Here's how the part is built. I have some questions about the finished solid (model axes, mm). A direction names the side the tool comes from. Coordinates: 2 decimals unless noted, no trailing zeros. Write each loop counter-clockwise with the first axis right and the second up, starting at its lowest first coordinate (ties: lowest second). Pieces come first, ordered by that corner, then holes. Notation, with made-up numbers: (-2.5, 84.25) - (1.5, 84.25) arc R20 cw to (1.5, 91.25) - close; hole circle Ø2 at (50.5, 71). An arc over 180 degrees is marked (long way). Answer in a Markdown table with one row per item. Add a question column.
Item 1: Imagine slicing it at B-B (z = -15). Please give me the cut outline in (x, y).
Item 2: We'd pull the mould along X, two halves only. Please class faces 5 (the face through (11, 37.369, -15)), 6 (the face through (30.322, 22, -15)), 7 (the face through (-22.678, 19, -17)): +X half, -X half, draft (parallel to the pull), parting line (faces both ways), or undercut.
Item 3: Which directions (+Z, -Z, +X, -X, +Y, -Y) give clear straight access to the entire face, cutting with the end or side of a thin tool? Please do faces 1 (the face through (25.322, 20, -17)), 2 (the face through (40, 6.369, -19)), 3 (the face through (-38, 6.369, -19)), 4 (the face through (-8.679, 33, -11)).
Item 4: Imagine slicing it at A-A (y = 31). Please give me the cut outline in (x, z).
Item 5: Imagine slicing it at D-D (x = 4). Please give me the cut outline in (y, z), plus the area to 3 significant figures.
Item 6: I'm going to push flat-ended pins straight in: pin 1 (5.5 mm diameter, centred on y = 25.5, z = -8.5, fed in from -X); pin 2 (12 mm diameter, centred on x = 16, y = 25.5, fed in from -Z); pin 3 (4.5 mm diameter, centred on x = 40.32, z = -15, fed in from +Y); pin 4 (7.5 mm diameter, centred on y = 16.5, z = -19.5, fed in from +X). Where does each tip first touch, or does it pass through?
Item 7: Imagine slicing it at C-C (y = 20.5). Please give me the cut outline in (x, z).
Item 8: If I drill on probe 1 along X at (y, z) = (31.5, -11); probe 2 along Y at (x, z) = (0.5, -22.5); probe 3 along Y at (x, z) = (-28, -25), over which ranges is the centre line in solid material (lowest first)? Write a range as from..to.
from build123d import *

# Parameters (mm, degrees)
F1_DEPTH = 30
F0_R     = 6.25
F2_DEPTH = 5
F3_W     = 5
F3_H     = 30
F4_DEPTH = 20
F5_W     = 5
F5_H     = 30
F6_DEPTH = 20
F7_R     = 2.5
F8_DEPTH = 25


# Not quite as in the source:
# - a feature names something its author has since deleted; it is built from what else it names


with BuildPart() as f1:
    # F0 (on Top) → F1 (new body)
    with BuildSketch(Plane.XY):
        Polygon((25.3224579843, 32.3690634753), (25.3224579843, 6.3690634753), (30.3224579843, 6.3690634753), (30.3224579843, 37.3690634753), (-8.6790506474, 37.3690634753), (-8.6790506474, 32.3690634753), align=None)
        Polygon((-22.6775420157, 6.3690634753), (-22.6775420157, 32.3690634753), (-21.1775420157, 32.3690634753), (-21.1775420157, 37.3690634753), (-27.6775420157, 37.3690634753), (-27.6775420157, 6.3690634753), align=None)
        Polygon((25.3224579843, 6.3690634753), (-22.6775420157, 6.3690634753), (-27.6775420157, 6.3690634753), (-27.6775420157, 1.3690634753), (30.3224579843, 1.3690634753), (30.3224579843, 6.3690634753), align=None)
    extrude(amount=-F1_DEPTH)

    # F0 (on Top) → F2 (join)
    with BuildSketch(Plane.XY):
        Polygon((-22.6775420157, 6.3690634753), (-22.6775420157, 32.3690634753), (-21.1775420157, 32.3690634753), (-21.1775420157, 37.3690634753), (-27.6775420157, 37.3690634753), (-27.6775420157, 6.3690634753), align=None)
        with BuildLine():
            Line((-21.1775420157, 32.3690634753), (-22.6775420157, 32.3690634753))
            Line((-22.6775420157, 32.3690634753), (-22.6775420157, 6.3690634753))
            Line((-22.6775420157, 6.3690634753), (25.3224579843, 6.3690634753))
            Line((25.3224579843, 6.3690634753), (25.3224579843, 32.3690634753))
            Line((25.3224579843, 32.3690634753), (-8.6790506474, 32.3690634753))
            Line((-8.6790506474, 32.3690634753), (-8.6790506474, 19.5063792474))
            ThreePointArc((-8.6790506474, 19.5063792474), (-14.858879986, 13.1194406446), (-21.1775420157, 19.3690634753))
            Line((-21.1775420157, 19.3690634753), (-21.1775420157, 32.3690634753))
        make_face()
        with Locations((6.6724579843, 19.3690634753)):
            Circle(F0_R, mode=Mode.SUBTRACT)
        Polygon((25.3224579843, 6.3690634753), (-22.6775420157, 6.3690634753), (-27.6775420157, 6.3690634753), (-27.6775420157, 1.3690634753), (30.3224579843, 1.3690634753), (30.3224579843, 6.3690634753), align=None)
        Polygon((25.3224579843, 32.3690634753), (25.3224579843, 6.3690634753), (30.3224579843, 6.3690634753), (30.3224579843, 37.3690634753), (-8.6790506474, 37.3690634753), (-8.6790506474, 32.3690634753), align=None)
    extrude(amount=-F2_DEPTH)

    # F3 (on face) → F4 (join)
    with BuildSketch(Plane.YZ.offset(30.3224579843)):
        with Locations((3.8690634753, -15)):
            Rectangle(F3_W, F3_H)
    extrude(amount=F4_DEPTH)

    # F5 (on face) → F6 (join)
    with BuildSketch(Plane(origin=(-27.6775420157, 0, 0), x_dir=(0, -1, 0), z_dir=(-1, 0, 0))):
        with Locations((-3.8690634753, -15)):
            Rectangle(F5_W, F5_H)
    extrude(amount=F6_DEPTH)

    # F7 (on face) → F8 (cut)
    with BuildSketch(Plane(origin=(0, 6.3690634753, 0), x_dir=(-1, 0, 0), z_dir=(0, 1, 0))):
        with Locations((-40.3224579843, -15)):
            Circle(F7_R)
        with Locations((37.6775420157, -15)):
            Circle(F7_R)
    extrude(amount=-F8_DEPTH, mode=Mode.SUBTRACT)


solid = f1.part
Here are the results:
| question | item | result |
|---|---|---|
| 1 | outline | (-47.68, 1.37) - (-40.18, 1.37) - (-40.18, 6.37) - (-47.68, 6.37) - close; (-35.18, 1.37) - (37.82, 1.37) - (37.82, 6.37) - (30.32, 6.37) - (30.32, 37.37) - (-8.68, 37.37) - (-8.68, 32.37) - (25.32, 32.37) - (25.32, 6.37) - (-22.68, 6.37) - (-22.68, 32.37) - (-21.18, 32.37) - (-21.18, 37.37) - (-27.68, 37.37) - (-27.68, 6.37) - (-35.18, 6.37) - close; (42.82, 1.37) - (50.32, 1.37) - (50.32, 6.37) - (42.82, 6.37) - close |
| 2 | face 5 | draft |
| 2 | face 6 | +X half |
| 2 | face 7 | undercut |
| 3 | face 1 | -Z |
| 3 | face 2 | +Z, -Z, +X, +Y |
| 3 | face 3 | +Z, -Z, -X, +Y |
| 3 | face 4 | +Z, -Z, +Y |
| 4 | outline | (-27.68, -30) - (-22.68, -30) - (-22.68, -5) - (-21.18, -5) - (-21.18, 0) - (-27.68, 0) - close; (-8.68, -5) - (25.32, -5) - (25.32, -30) - (30.32, -30) - (30.32, 0) - (-8.68, 0) - close |
| 5 | outline | (1.37, -30) - (6.37, -30) - (6.37, -5) - (13.72, -5) - (13.72, 0) - (1.37, 0) - close; (25.02, -5) - (32.37, -5) - (32.37, -30) - (37.37, -30) - (37.37, 0) - (25.02, 0) - close |
| 5 | area | 374 mm2 |
| 6 | pin 1 | stops at x = -27.68 |
| 6 | pin 2 | stops at z = -5 |
| 6 | pin 3 | passes through |
| 6 | pin 4 | stops at x = 30.32 |
| 7 | outline | (-27.68, -30) - (-22.68, -30) - (-22.68, -5) - (-21.18, -5) - (-21.18, 0) - (-27.68, 0) - close; (-8.68, -5) - (0.53, -5) - (0.53, 0) - (-8.68, 0) - close; (12.82, -5) - (25.32, -5) - (25.32, -30) - (30.32, -30) - (30.32, 0) - (12.82, 0) - close |
| 8 | probe 1 | x = -27.68..-22.68, 25.32..30.32 |
| 8 | probe 2 | y = 1.37..6.37, 32.37..37.37 |
| 8 | probe 3 | y = 1.37..6.37 |
